For this review, use the dimensioned drawing (mm, ordinates from the lowest corner) and the shaded views. A direction names the side the tool comes from. Give positions to 0.01 mm unless a question says otherwise; leave off trailing zeros. Loops run counter-clockwise (first coordinate to the right, second up) from the corner with the lowest first, then second, coordinate; pieces in that order, holes last. Notation, with made-up numbers: M 7.5,-15 L 47.5,-15 A20 ccw 47.5,24 Z; hole C 78.5,0 d2. An arc over 180 degrees is marked long. Use CSV: the item, a comma, the result in double quotes. Start each with the question number.
1. To check wall thickness, follow line 1 (Z direction, x = 14.75, y = 6); line 2 (Y direction, x = 10.25, z = 12.75); line 3 (Z direction, x = 5.25, y = 10). State the ranges of each line that lie inside material, in increasing order. Write a range as [from, to].
2. Take a section at D-D, the plane y = 6.35. State how many separate pieces and enclosed holes the cut face has.
3. Take a section at C-C, the plane x = 12.75. Write out the cut boundary in (y, z), and give its area (3 significant figures).
4. Take a section at B-B, the plane y = 1.75. Write out the cut boundary in (x, z).
5. Tool access review of the marked faces 4, 5 and 6: name each direction out of +Z, -Z, +X, -X, +Y, -Y from which nothing blocks a thin tool from reaching the whole face with its end or side.
6. Insertion check: P1, Ø4, axis at x = 9, z = 11, coming from the -Y side; P2, Ø1.5, axis at x = 7.5, z = 1.5, coming from the -Y side; P3, Ø6, axis at x = 13.5, y = 3, coming from the -Z side; P4, Ø2.5, axis at x = 10, z = 2, coming from the -Y side (3 decimals). Each pin has a flat end and moves straight along its axis. Give the tip position at first contact, or say it passes through.
7. The part is to be moulded in two halves that separate along Z. For the marked faces 1, 2 and 3, say which applies: pulls with the +Z half, pulls with the -Z half, needs draft (parallel to the pull), parting line crosses it, or undercut.
8. Take a section at A-A, the plane z = 14. Write out the cut boundary in (x, y).
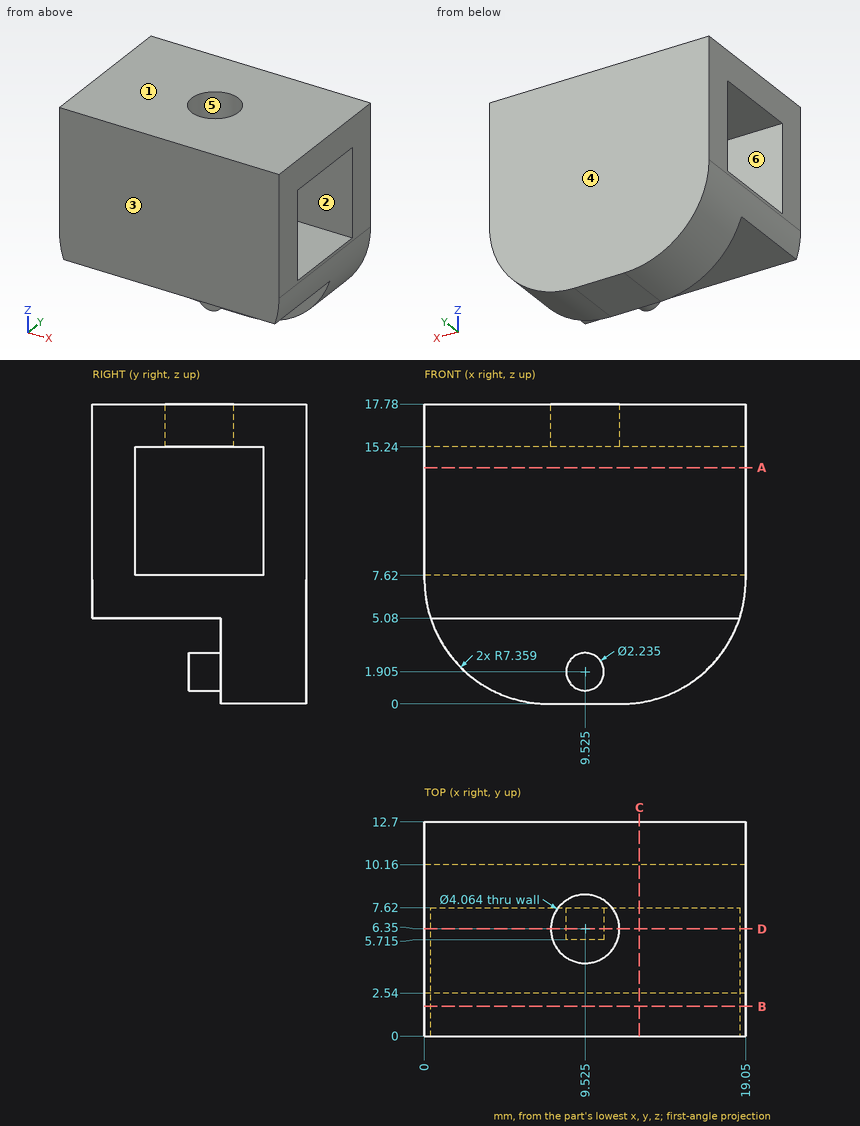
Result set:
1,line 1,"[5.08, 7.62], [15.24, 17.78]"
1,line 2,"[0, 2.54], [10.16, 12.7]"
1,line 3,"[0.31, 7.62], [15.24, 17.78]"
2,separate pieces,"4"
2,enclosed holes,"0"
3,outline,"M 0,5.08 L 7.62,5.08 L 7.62,0.08 L 12.7,0.08 L 12.7,17.78 L 0,17.78 Z; hole M 2.54,7.62 L 10.16,7.62 L 10.16,15.24 L 2.54,15.24 Z"
3,area,"129 mm2"
4,outline,"M 0,7.36 A7.36 ccw 0.36,5.08 L 18.69,5.08 A7.36 ccw 19.05,7.36 L 19.05,17.78 L 0,17.78 Z"
5,face 4,"+Z, -Z, +X, -X, +Y"
5,face 5,"+Z"
5,face 6,"+X, -X"
6,P1,"y = 0"
6,P2,"y = 7.62"
6,P3,"z = 5.08"
6,P4,"y = 5.715"
7,face 1,"pulls with the +Z half"
7,face 2,"undercut"
7,face 3,"needs draft"
8,outline,"M 0,0 L 19.05,0 L 19.05,2.54 L 0,2.54 Z; M 0,10.16 L 19.05,10.16 L 19.05,12.7 L 0,12.7 Z"
